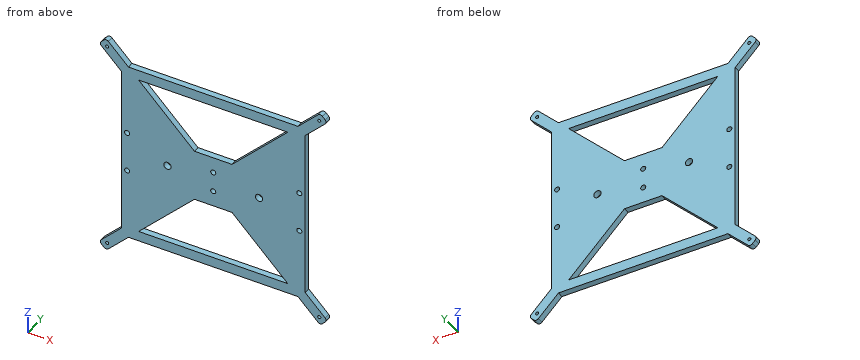
```python
from build123d import *

# Parameters (mm, degrees)
BOSS_EXTRUDE2_DEPTH = 6
SKETCH1_6_R         = 1.55
CUT_EXTRUDE4_DEPTH  = 6
SKETCH2_R           = 2.5
SKETCH2_R_2         = 3.6
CUT_EXTRUDE5_DEPTH  = 6
SKETCH3_R           = 2.5
CUT_EXTRUDE6_DEPTH  = 6
CUT_EXTRUDE7_DEPTH  = 6


with BuildPart() as part:
    # Sketch1 → Boss-Extrude2 (new body)
    with BuildSketch(Plane(origin=(0, 0, 0), x_dir=(1, 0, 0), z_dir=(0, 1, 0))):
        with BuildLine():
            Line((-83.5, 90.571067812), (83.5, 90.571067812))
            Line((83.5, 90.571067812), (103.298989873, 110.370057685))
            ThreePointArc((103.298989873, 110.370057685), (105.420310217, 111.248737342), (107.54163056, 110.370057685))
            Line((107.54163056, 110.370057685), (110.370057685, 107.54163056))
            ThreePointArc((110.370057685, 107.54163056), (111.248737342, 105.420310217), (110.370057685, 103.298989873))
            Line((110.370057685, 103.298989873), (90.571067812, 83.5))
            Line((90.571067812, 83.5), (90.571067812, -83.5))
            Line((90.571067812, -83.5), (110.370057685, -103.298989873))
            ThreePointArc((110.370057685, -103.298989873), (111.248737342, -105.420310217), (110.370057685, -107.54163056))
            Line((110.370057685, -107.54163056), (107.54163056, -110.370057685))
            ThreePointArc((107.54163056, -110.370057685), (105.420310217, -111.248737342), (103.298989873, -110.370057685))
            Line((103.298989873, -110.370057685), (83.5, -90.571067812))
            Line((83.5, -90.571067812), (-83.5, -90.571067812))
            Line((-83.5, -90.571067812), (-103.298989873, -110.370057685))
            ThreePointArc((-103.298989873, -110.370057685), (-105.420310217, -111.248737342), (-107.54163056, -110.370057685))
            Line((-107.54163056, -110.370057685), (-110.370057685, -107.54163056))
            ThreePointArc((-110.370057685, -107.54163056), (-111.248737342, -105.420310217), (-110.370057685, -103.298989873))
            Line((-110.370057685, -103.298989873), (-90.571067812, -83.5))
            Line((-90.571067812, -83.5), (-90.571067812, 83.5))
            Line((-90.571067812, 83.5), (-110.370057685, 103.298989873))
            ThreePointArc((-110.370057685, 103.298989873), (-111.248737342, 105.420310217), (-110.370057685, 107.54163056))
            Line((-110.370057685, 107.54163056), (-107.54163056, 110.370057685))
            ThreePointArc((-107.54163056, 110.370057685), (-105.420310217, 111.248737342), (-103.298989873, 110.370057685))
            Line((-103.298989873, 110.370057685), (-83.5, 90.571067812))
        make_face()
    extrude(amount=BOSS_EXTRUDE2_DEPTH)

    # Sketch1<6> → Cut-Extrude4 (cut)
    with BuildSketch(Plane(origin=(0, 0, 0), x_dir=(1, 0, 0), z_dir=(0, 1, 0))):
        with Locations((-104.5, 104.5)):
            Circle(SKETCH1_6_R)
        with Locations((104.5, 104.5)):
            Circle(SKETCH1_6_R)
        with Locations((104.5, -104.5)):
            Circle(SKETCH1_6_R)
        with Locations((-104.5, -104.5)):
            Circle(SKETCH1_6_R)
    extrude(amount=CUT_EXTRUDE4_DEPTH, mode=Mode.SUBTRACT)

    # Sketch2 → Cut-Extrude5 (cut)
    with BuildSketch(Plane(origin=(0, 6, 0), x_dir=(1, 0, 0), z_dir=(0, 1, 0))):
        with Locations((-84.85, 20)):
            Circle(SKETCH2_R)
        with Locations((-84.85, -20)):
            Circle(SKETCH2_R)
        with Locations((45.15, 0)):
            Circle(SKETCH2_R_2)
        with Locations((84.85, -20)):
            Circle(SKETCH2_R)
        with Locations((-45.15, 0)):
            Circle(SKETCH2_R_2)
        with Locations((84.85, 20)):
            Circle(SKETCH2_R)
    extrude(amount=-CUT_EXTRUDE5_DEPTH, mode=Mode.SUBTRACT)

    # Sketch3 → Cut-Extrude6 (cut)
    with BuildSketch(Plane(origin=(0, 6, 0), x_dir=(1, 0, 0), z_dir=(0, 1, 0))):
        with Locations((0, 10)):
            Circle(SKETCH3_R)
        with Locations((0, -10)):
            Circle(SKETCH3_R)
    extrude(amount=-CUT_EXTRUDE6_DEPTH, mode=Mode.SUBTRACT)

    # Sketch4 → Cut-Extrude7 (cut)
    with BuildSketch(Plane(origin=(0, 6, 0), x_dir=(1, 0, 0), z_dir=(0, 1, 0))):
        Polygon((-73.5, 80.571067812), (73.5, 80.571067812), (18.5, 25.571067812), (-18.5, 25.571067812), align=None)
        Polygon((73.5, -80.571067812), (18.5, -25.571067812), (-18.5, -25.571067812), (-73.5, -80.571067812), align=None)
    extrude(amount=-CUT_EXTRUDE7_DEPTH, mode=Mode.SUBTRACT)


solid = part.part
```
Part model, mm, in its own coordinate system. Round coordinates to 2 decimals unless told otherwise and drop trailing zeros. Loops run counter-clockwise (first coordinate to the right, second up) from the corner with the lowest first, then second, coordinate; pieces in that order, holes last. Notation, with made-up numbers: (-19.75, 63) -> (-15.75, 63) arc R18 cw to (-15.75, 88) -> close; hole circle Ø9 at (79.25, 8). An arc over 180 degrees is marked (long way). Use a Markdown table: item, result.
1) Cut at C-C, the plane x = 45.15. List the corners of the cut face in (y, z).
The answers:
| item | result |
|---|---|
| outline | (0, -90.57) -> (6, -90.57) -> (6, -80.57) -> (0, -80.57) -> close; (0, -52.22) -> (6, -52.22) -> (6, -3.6) -> (0, -3.6) -> close; (0, 3.6) -> (6, 3.6) -> (6, 52.22) -> (0, 52.22) -> close; (0, 80.57) -> (6, 80.57) -> (6, 90.57) -> (0, 90.57) -> close |
2) Cut at B-B, the plane z = 44.5. List the corners of the cut face in (x, y), and give its area (3 significant figures).
The answers:
| item | result |
|---|---|
| outline | (-90.57, 0) -> (-37.43, 0) -> (-37.43, 6) -> (-90.57, 6) -> close; (37.43, 0) -> (90.57, 0) -> (90.57, 6) -> (37.43, 6) -> close |
| area | 638 mm2 |
3) Cut at A-A, the plane x = -9. List the corners of the cut face in (y, z).
The answers:
| item | result |
|---|---|
| outline | (0, -90.57) -> (6, -90.57) -> (6, -80.57) -> (0, -80.57) -> close; (0, -25.57) -> (6, -25.57) -> (6, 25.57) -> (0, 25.57) -> close; (0, 80.57) -> (6, 80.57) -> (6, 90.57) -> (0, 90.57) -> close |
4) Drop flat-ended pins along their axis: pin 1 Ø1.9 at (x, z) = (104.5, -104.5) entering from +Y (3 decimals); pin 2 Ø1.8 at (x, y) = (-17, 3.5) entering from -Z; pin 3 Ø1.5 at (x, y) = (3.5, 0.5) entering from +Z; pin 4 Ø2 at (y, z) = (1.5, -62) entering from +X. Give the stop position or say it passes through.
The answers:
| item | result |
|---|---|
| pin 1 | passes through |
| pin 2 | stops at z = -90.57 |
| pin 3 | stops at z = 90.57 |
| pin 4 | stops at x = 90.57 |
5) Cut at D-D, the plane y = 3.8. State how many separate pieces and enclosed holes the cut face has, and give its area (3 significant figures).
The answers:
| item | result |
|---|---|
| separate pieces | 1 |
| enclosed holes | 14 |
| area | 23,600 mm2 |
6) Probe line 1 (Z direction, x = 0, y = 4.7); line 2 (X direction, y = 2.2, z = -20); line 3 (Z direction, x = 32.5, y = 2.7). List the from-to ranges inside material, lowest first. Write a range as [from, to].
The answers:
| item | result |
|---|---|
| line 1 | z = [-90.57, -80.57], [-25.57, -12.5], [-7.5, 7.5], [12.5, 25.57], [80.57, 90.57] |
| line 2 | x = [-90.57, -87.35], [-82.35, 82.35], [87.35, 90.57] |
| line 3 | z = [-90.57, -80.57], [-39.57, 39.57], [80.57, 90.57] |
